The model under review builds one solid part; all positions refer to its coordinate system, in mm. A direction names the side the tool comes from. Give positions to 0.01 mm unless a question says otherwise; leave off trailing zeros. Loops run counter-clockwise (first coordinate to the right, second up) from the corner with the lowest first, then second, coordinate; pieces in that order, holes last. Notation, with made-up numbers: M 43.25,2 L 54.25,2 A4 ccw 54.25,6 Z; hole C 7.5,-31 d10. An arc over 180 degrees is marked long. Write item = value, one per line. Start each with the question number.
1. Draft analysis for pull direction Z (two halves, no side actions). For faces 4 (the face through (0, -53, -12.5)), 5 (the face through (-1, -55, 0)), 6 (the face through (-63, -50, 10)), 7 (the face through (-80, -52.5, 0)), state which applies: pulls with the +Z half, pulls with the -Z half, needs draft (parallel to the pull), parting line crosses it, or undercut.
2. For pin 1 (1 mm diameter, centred on x = 20, z = 2, fed in from +Y); pin 2 (1 mm diameter, centred on y = -4.5, z = -8.5, fed in from +X); pin 3 (10 mm diameter, centred on y = -33.5, z = 1.5, fed in from -X), all flat-tipped, find the tip position at first contact; note any pin that passes through.
3. We need section C-C on z = 6.5. Give the boundary of the cut face in (x, y).
4. We need section D-D on y = 5. Give the boundary of the cut face in (x, z), then the cut area to 3 significant figures.
5. For faces 1 (the face through (80, -52.5, 0)), 2 (the face through (-63, -50, -10)), 3 (the face through (1, -52.5, 0)), list the 3-axis set-ups (+Z, -Z, +X, -X, +Y, -Y) from which the entire face can be reached by the end or side of a thin tool; tool diameter is ignored.
6. We need section A-A on y = -45. Give the boundary of the cut face in (x, z).
7. We need section B-B on x = 63. Give the boundary of the cut face in (y, z), then the cut area to 3 significant figures.
8. Wall thickness on line 1 along X through (y, z) = (-25.5, 5.5); line 2 along Y through (x, z) = (-44, 1.5); line 3 along Y through (x, z) = (67, -11.5): over which ranges is each line inside the solid? List them lowest first. Write a range as from..to.
Autodesk Inventor part; units mm, degrees
ref_plane "YZ Plane" through (0, 0, 0) normal (1, 0, 0) x (0, 1, 0)
ref_plane "XZ Plane" through (0, 0, 0) normal (0, 1, 0) x (-1, 0, 0)
ref_plane "XY Plane" through (0, 0, 0) normal (0, 0, 1) x (1, 0, 0)
sketch "Sketch1" plane through (0, 0, 0) normal (0, 0, 1) x (1, 0, 0)
  line L0 (-60, 52.5) -> (60, 52.5)
  line L1 (60, 52.5) -> (60, -52.5)
  line L2 (60, -52.5) -> (-60, -52.5)
  line L3 (-60, -52.5) -> (-60, 52.5)
  line L4 (-60, 52.5) -> (60, -52.5) construction
  line L5 (60, 52.5) -> (-60, -52.5) construction
  circle A0 centre (0, 0) radius 52.5
  line L6 (-52.5, 0) -> (-60, 0)
  line L7 (52.5, 0) -> (60, 0)
  line L8 (-100, -55) -> (100, -55)
  line L9 (100, -55) -> (100, -50)
  line L10 (100, -50) -> (-100, -50)
  line L11 (-100, -50) -> (-100, -55)
  line L12 (-100, -55) -> (100, -50) construction
  line L13 (100, -55) -> (-100, -50) construction
  line L14 (-57.5, 52.5) -> (57.5, 52.5)
  line L15 (57.5, 52.5) -> (57.5, -52.5)
  line L16 (57.5, -52.5) -> (-57.5, -52.5)
  line L17 (-57.5, -52.5) -> (-57.5, 52.5)
  line L18 (-57.5, 52.5) -> (57.5, -52.5) construction
  line L19 (57.5, 52.5) -> (-57.5, -52.5) construction
  line L20 (-100, -52.5) -> (100, -52.5)
  point P0 (0, -52.5)
  point P1 (-60, -50)
  point P2 (60, -50)
  point P3 (60, -52.5)
  point P4 (57.5, 52.5)
  point P5 (57.5, -52.5)
  point P6 (-57.5, 52.5)
  point P7 (-60, -52.5)
  dimension "d0" = 120
  dimension "d1" = 105
  dimension "d2" = 105
  dimension "d5" = 200
  dimension "d6" = 5
  dimension "d30" = 115
  dimension "d31" = 105
extrude "Extrusion1" add sketch "Sketch1" along normal mid plane 25 contours L0 L17 L6 L3 | L6 L17 L10 L3 | L10 L17 L2 L3 | L0 L1 L7 L15 | L2 L20 L9 L8 L11 | L7 L1 L10 L15 | L10 L1 L2 L15
sketch "Sketch6" plane through (0, 0, 12.5) normal (0, 0, 1) x (1, 0, 0)
  line L0 (-60, -52.5) -> (-60, -42.5)
  line L1 (-60, 52.5) -> (-60, -52.5)
  line L2 (-60, -52.5) -> (-70, -52.5)
  line L3 (-60, -52.5) -> (-100, -52.5)
  line L4 (-70, -52.5) -> (-60, -42.5)
  line L5 (0, -52.5) -> (0, -39.6875)
  line L6 (60, -52.5) -> (60, -42.5)
  line L7 (60, -52.5) -> (70, -52.5)
  line L8 (70, -52.5) -> (60, -42.5)
  point P0 (0, 0)
  dimension "d32" = 10
  dimension "d33" = 10
extrude "Extrusion5" add sketch "Sketch6" against normal blind 2.5
mirror "Mirror1" about plane through (0, 0, 0) normal (0, 0, 1) of "Extrusion5"
properties part number "SOPORTE DE GUIA"
Final values:
q1.face_4 = pulls with the -Z half
q1.face_5 = needs draft
q1.face_6 = undercut
q1.face_7 = undercut
q2.pin_1 = -52.5
q2.pin_2 = 60
q2.pin_3 = -60
q3.outline = M -100,-55 L 100,-55 L 100,-52.5 L 60,-52.5 L 60,52.5 L 57.5,52.5 L 57.5,-52.5 L -57.5,-52.5 L -57.5,52.5 L -60,52.5 L -60,-52.5 L -100,-52.5 Z
q4.outline = M -60,-12.5 L -57.5,-12.5 L -57.5,12.5 L -60,12.5 Z; M 57.5,-12.5 L 60,-12.5 L 60,12.5 L 57.5,12.5 Z
q4.area = 125 mm²
q5.face_1 = +X, +Y
q5.face_2 = -X, +Y
q5.face_3 = +Z, -Z, +Y
q6.outline = M -62.5,-12.5 L -57.5,-12.5 L -57.5,12.5 L -62.5,12.5 L -62.5,10 L -60,10 L -60,-10 L -62.5,-10 Z; M 57.5,-12.5 L 62.5,-12.5 L 62.5,-10 L 60,-10 L 60,10 L 62.5,10 L 62.5,12.5 L 57.5,12.5 Z
q7.outline = M -55,-12.5 L -45.5,-12.5 L -45.5,-10 L -52.5,-10 L -52.5,10 L -45.5,10 L -45.5,12.5 L -55,12.5 Z
q7.area = 97.5 mm²
q8.line_1 = -60..-57.5, 57.5..60
q8.line_2 = -55..-52.5
q8.line_3 = -55..-49.5
